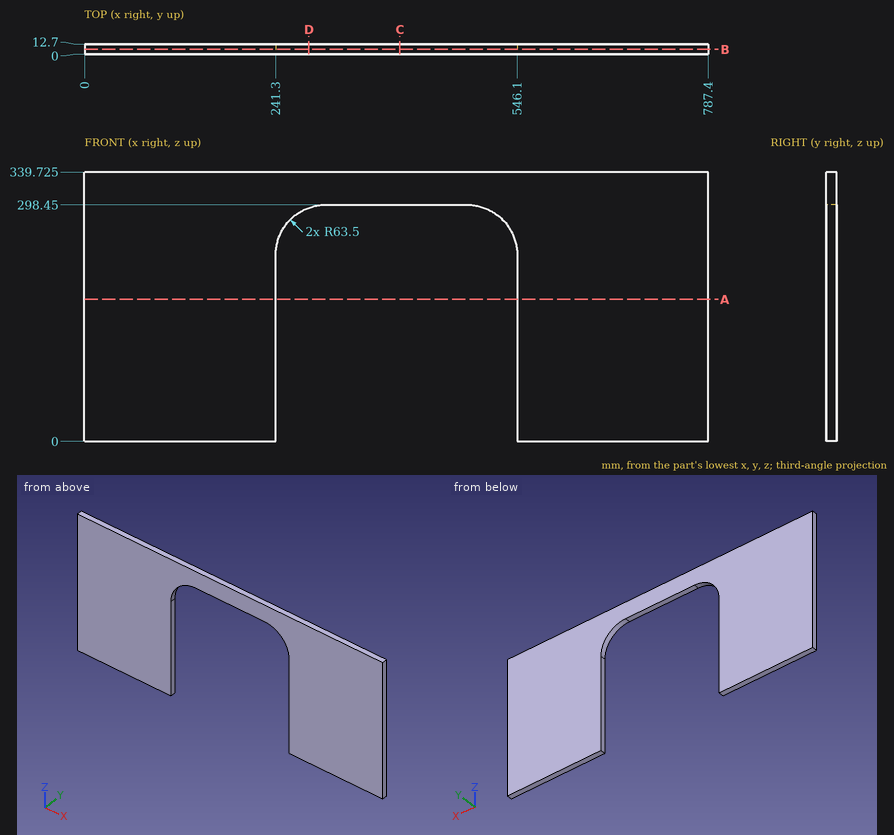
Source: three-view drawing plus pictorial views. Frame: mm from the lowest corner of the part. Give positions to 0.01 mm unless a question says otherwise; leave off trailing zeros. Write each loop counter-clockwise with the first axis right and the second up, starting at its lowest first coordinate (ties: lowest second). Pieces come first, ordered by that corner, then holes. Notation, with made-up numbers: (-14.5, 49.25) -> (4.5, 49.25) arc R20 ccw to (4.5, 60.25) -> close; hole circle Ø5 at (71, 67.25). An arc over 180 degrees is marked (long way). Answer in a Markdown table with one row per item.
(1) Pin query (flat end, axial travel): pin 1 (1.5 mm diameter, centred on x = 495, z = 304.5, fed in from -Y); pin 2 (4 mm diameter, centred on x = 385, y = 7.5, fed in from -Z). Return the tip coordinate at first contact, or that it passes through.
Answers below:
| item | result |
|---|---|
| pin 1 | y = 0 |
| pin 2 | z = 298.45 |
(2) Section query D-D on x = 283. Return loops of the section in (y, z) (3 decimals).
Answers below:
| item | result |
|---|---|
| outline | (0, 294.591) -> (12.7, 294.591) -> (12.7, 339.725) -> (0, 339.725) -> close |
(3) Section query A-A on z = 179. Return loops of the section in (x, y).
Answers below:
| item | result |
|---|---|
| outline | (0, 0) -> (241.3, 0) -> (241.3, 12.7) -> (0, 12.7) -> close; (546.1, 0) -> (787.4, 0) -> (787.4, 12.7) -> (546.1, 12.7) -> close |
(4) Section query C-C on x = 398. Return loops of the section in (y, z) (3 decimals), then the cut area to 3 significant figures.
Answers below:
| item | result |
|---|---|
| outline | (0, 298.45) -> (12.7, 298.45) -> (12.7, 339.725) -> (0, 339.725) -> close |
| area | 524 mm^2 |
(5) Section query B-B on y = 6. Return loops of the section in (x, z) (3 decimals), then the cut area to 3 significant figures.
Answers below:
| item | result |
|---|---|
| outline | (0, 0) -> (241.3, 0) -> (241.3, 234.95) arc R63.5 cw to (304.8, 298.45) -> (482.6, 298.45) arc R63.5 cw to (546.1, 234.95) -> (546.1, 0) -> (787.4, 0) -> (787.4, 339.725) -> (0, 339.725) -> close |
| area | 178,000 mm^2 |
(6) Ray query, line 1 along X through (y, z) = (4, 181.5); line 2 along X through (y, z) = (3, 260.5); line 3 along Z through (x, y) = (396, 6) (3 decimals). Return the intervals inside material, ascending. Write a range as [from, to].
Answers below:
| item | result |
|---|---|
| line 1 | [0, 241.3], [546.1, 787.4] |
| line 2 | [0, 246.67], [540.73, 787.4] |
| line 3 | [298.45, 339.725] |
